Study the drawing (mm; zero at the part's minimum x, y, z) and answer. A direction names the side the tool comes from. Round coordinates to 2 decimals unless told otherwise and drop trailing zeros. Order: outer loops, then holes, each group sorted by start corner. A loop starts at its lowest first (then second) coordinate and runs counter-clockwise, first axis right, second up. Notation, with made-up numbers: (-13.75, -1.75) - (25.25, -1.75) arc R30 ccw to (25.25, 28.25) - close; hole circle Ø2 at (40, 13). An arc over 180 degrees is marked (long way). Use one line per item in the form item = value. Start each with the question number.
Q1. Which of the six approach directions +Z, -Z, +X, -X, +Y, -Y give full straight-line access (tool end or side, diameter ignored) to the marked faces 1, 2 and 3?
Q2. For a pull along Y with two mould halves and no side action, classify the marked faces 4, 5 and 6 as +Y half, -Y half, draft (parallel to the pull), parting line (faces both ways), or undercut.
Q3. The part is cut by section A-A on x = 11. Determine the outline of the cut face in (y, z), plus the area to 3 significant figures.
Q4. The part is cut by section D-D on x = 53.5. Determine the outline of the cut face in (y, z).
Q5. The part is cut by section C-C on z = 8.5. Determine the outline of the cut face in (x, y).
Q6. Find the intervals of material crossed by line 1 (X direction, y = 51.5, z = 4.5); line 2 (Y direction, x = 7, z = 2); line 3 (Z direction, x = 74, y = 29), in increasing order. Write a range as [from, to].
Q7. The part is cut by section B-B on y = 25.5. Determine the outline of the cut face in (x, z).
Q8. Given P1, Ø1.6, axis at x = 13, z = 14, coming from the -Y side; P2, Ø6, axis at x = 73.5, y = 26, coming from the -Z side; P3, Ø8, axis at y = 28, z = 6, coming from the -X side; P4, Ø6, axis at x = 43, z = 4.5, coming from the -Y side, each flat-ended and moving along its own axis, determine where each tip first touches the part or whether it passes through.
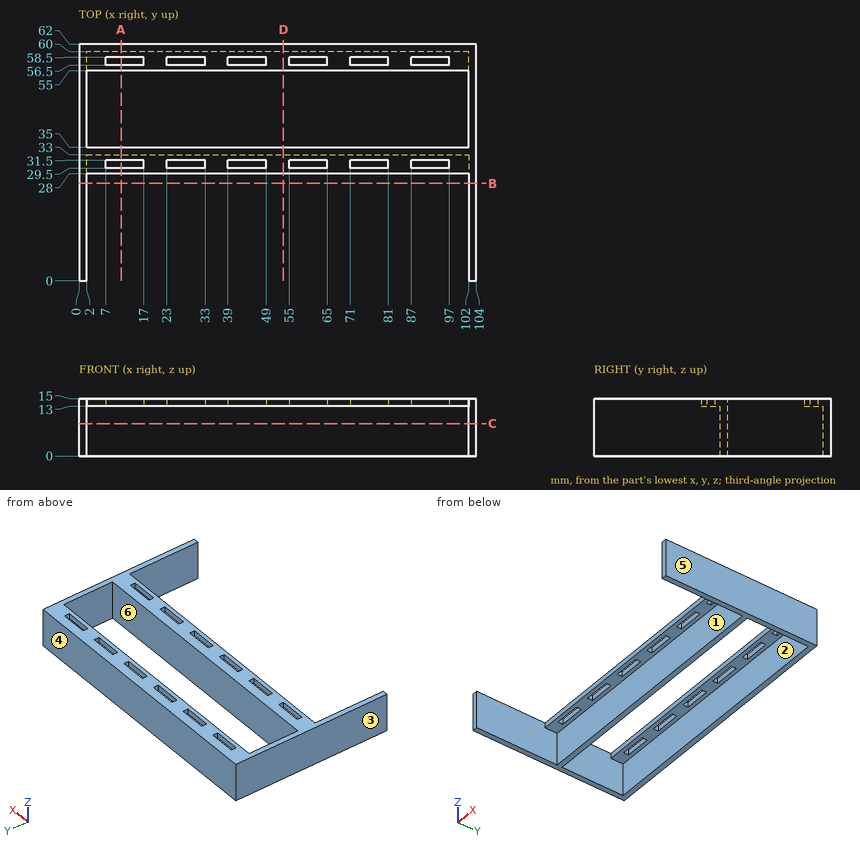
Found:
q1.face_1 = -Z, -Y
q1.face_2 = -Z
q1.face_3 = +Z, -Z, -X, +Y, -Y
q2.face_4 = +Y half
q2.face_5 = draft
q2.face_6 = undercut
q3.outline = (28, 13) - (29.5, 13) - (29.5, 15) - (28, 15) - close; (31.5, 13) - (33, 13) - (33, 0) - (35, 0) - (35, 15) - (31.5, 15) - close; (55, 13) - (56.5, 13) - (56.5, 15) - (55, 15) - close; (58.5, 13) - (60, 13) - (60, 0) - (62, 0) - (62, 15) - (58.5, 15) - close
q3.area = 72.0 mm²
q4.outline = (28, 13) - (33, 13) - (33, 0) - (35, 0) - (35, 15) - (28, 15) - close; (55, 13) - (60, 13) - (60, 0) - (62, 0) - (62, 15) - (55, 15) - close
q5.outline = (0, 0) - (2, 0) - (2, 33) - (102, 33) - (102, 0) - (104, 0) - (104, 62) - (0, 62) - close; hole (2, 35) - (102, 35) - (102, 60) - (2, 60) - close
q6.line_1 = [0, 2], [102, 104]
q6.line_2 = [33, 35], [60, 62]
q6.line_3 = [13, 15]
q7.outline = (0, 0) - (2, 0) - (2, 15) - (0, 15) - close; (102, 0) - (104, 0) - (104, 15) - (102, 15) - close
q8.P1 = 28
q8.P2 = 13
q8.P3 = 0
q8.P4 = 33
